Check sheet for the modelled part. Datum: model origin and axes. Units: mm. Coordinates: 2 decimals unless noted, no trailing zeros. Order: outer loops, then holes, each group sorted by start corner. A loop starts at its lowest first (then second) coordinate and runs counter-clockwise, first axis right, second up.
1. Draft check along Z on faces 1 (the cylindrical face through (13.49, 0.19, 10.89)), 2 (the cylindrical face through (-9.643, 0.188, -10.567)), 3 (the flat face through (0, 0.381, 0)). Enter one of: released by +Z, released by -Z, zero draft, split by the parting line, or undercut.
2. Cross-section at B-B (y = 0.1). Enter the section's corners in (x, z).
3. Thickness scan on line 1 (X direction, y = 0.2, z = -7); line 2 (X direction, y = 0.15, z = -7.5); line 3 (Z direction, x = 12.5, y = 0.2). Record the ranges inside material, lowest first.
4. Gauge pin test, flat ends, axial feed: pin 1 Ø1.3 at (x, z) = (13.81, 0) entering from -Y; pin 2 Ø3 at (x, z) = (-11, 6) entering from -Y. Record the tip position at first contact, or that the pin passes through.
5. Cross-section at A-A (z = 0). Enter the section's corners in (x, y), then the cut area to 3 significant figures.
6. Cross-section at C-C (z = -9). Enter the section's corners in (x, y), then the cut area to 3 significant figures.
```python
from build123d import *

# Parameters (mm, degrees)
SKETCH1_W                 = 30.7975
SKETCH1_H                 = 25.4
BOSS_EXTRUDE1_DEPTH       = 0.381
FILLET1_R                 = 6.35
F_0_CLEARANCE_HOLE1_D     = 1.6129
F_0_CLEARANCE_HOLE1_DEPTH = 25.4
F_0_CLEARANCE_HOLE1_TIP   = 0.484564046


with BuildPart() as part:
    # Sketch1 → Boss-Extrude1 (new body)
    with BuildSketch(Plane(origin=(0, 0, 0), x_dir=(1, 0, 0), z_dir=(0, 1, 0))):
        Rectangle(SKETCH1_W, SKETCH1_H)
    extrude(amount=BOSS_EXTRUDE1_DEPTH)

    # Fillet1
    fillet1_edges = [part.edges().sort_by_distance(p)[0] for p in [
        (15.39875, 0.1905, 12.7),
        (15.39875, 0.1905, -12.7),
    ]]
    fillet(fillet1_edges, radius=FILLET1_R)

    # #0 Clearance Hole1
    with Locations(Plane(origin=(0, 0.381, 0), x_dir=(-1, 0, 0), z_dir=(0, 1, 0))):
        with Locations((9.04875, -11.1125), (-3.65125, -11.1125), (-13.81125, 0), (9.04875, 11.1125), (-3.65125, 11.1125)):
            Hole(F_0_CLEARANCE_HOLE1_D / 2, depth=F_0_CLEARANCE_HOLE1_DEPTH)
            with Locations((0, 0, -(F_0_CLEARANCE_HOLE1_DEPTH + F_0_CLEARANCE_HOLE1_TIP / 2))):  # 118° drill point
                Cone(0, F_0_CLEARANCE_HOLE1_D / 2, F_0_CLEARANCE_HOLE1_TIP, mode=Mode.SUBTRACT)


solid = part.part
```
Data:
1. face 1: released by +Z
1. face 2: undercut
1. face 3: zero draft
2. outline: (-15.4, -12.7) - (9.05, -12.7) arc R6.35 ccw to (15.4, -6.35) - (15.4, 6.35) arc R6.35 ccw to (9.05, 12.7) - (-15.4, 12.7) - close; hole circle Ø1.61 at (-9.05, -11.11); hole circle Ø1.61 at (-9.05, 11.11); hole circle Ø1.61 at (3.65, -11.11); hole circle Ø1.61 at (3.65, 11.11); hole circle Ø1.61 at (13.81, 0)
3. line 1: x = -15.4 to 15.37
3. line 2: x = -15.4 to 15.29
3. line 3: z = -11.68 to 11.68
4. pin 1: passes through
4. pin 2: stops at y = 0
5. outline: (-15.4, 0) - (13, 0) - (13, 0.38) - (-15.4, 0.38) - close; (14.62, 0) - (15.4, 0) - (15.4, 0.38) - (14.62, 0.38) - close
5. area: 11.1 mm2
6. outline: (-15.4, 0) - (14.82, 0) - (14.82, 0.38) - (-15.4, 0.38) - close
6. area: 11.5 mm2
